Model file for the job. Use its own axes, mm. Face numbers are marked on the shaded views. A direction names the side the tool comes from. Give positions to 0.01 mm unless a question says otherwise; leave off trailing zeros. Write each loop counter-clockwise with the first axis right and the second up, starting at its lowest first coordinate (ties: lowest second). Pieces come first, ordered by that corner, then holes. Notation, with made-up numbers: (46, -25.5) - (53, -25.5) arc R18 ccw to (53, -7.5) - close; hole circle Ø10 at (31, 16.25). An arc over 180 degrees is marked (long way). One line per item, written item: value. Start each with the question number.
(1) Drop flat-ended pins along their axis: P1, Ø12, axis at y = 300, z = -22.5, coming from the -X side; P2, Ø4, axis at x = -13.5, z = -37, coming from the -Y side; P3, Ø3.5, axis at x = -26.99, z = -26.99, coming from the -Y side (1 decimal); P4, Ø12, axis at x = -19.5, z = -29.5, coming from the -Y side. Give the stop position or say it passes through.
(2) Cut at B-B, the plane y = 261. List the corners of the cut face in (x, z) (1 decimal).
(3) Cut at A-A, the plane y = 227. List the corners of the cut face in (x, z) (1 decimal).
(4) 3-axis set-ups, long thin cutter, end or side, ignore diameter. For the marked faces 1 and 2: which of +Z, -Z, +X, -X, +Y, -Y reach the whole face in a straight line?
(5) Cut at C-C, the plane x = -5. List the corners of the cut face in (y, z) (3 decimals), and give its area (3 significant figures).
(6) Probe L1, parallel to Y at x = -23.5, z = -38; L2, parallel to X at y = 248.5, z = -28.5; L3, parallel to Z at x = -28, y = 237. List the from-to ranges inside material, lowest first.
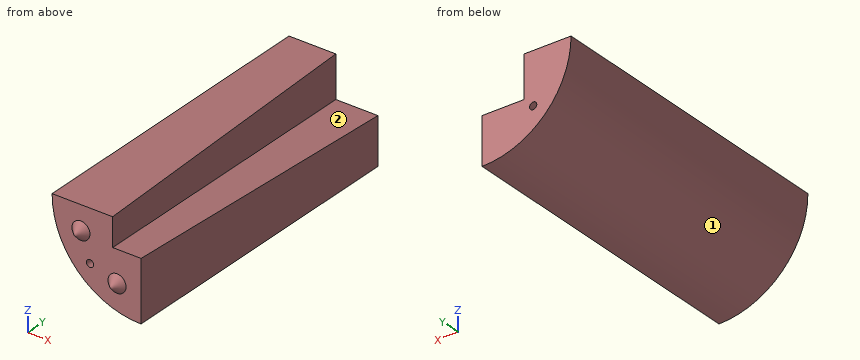
from build123d import *

# Parameters (mm, degrees)
SKETCH1_R           = 46.99
BOSS_EXTRUDE1_DEPTH = 330.2
SKETCH2_W           = 44.45
SKETCH2_H           = 44.45
CUT_EXTRUDE1_DEPTH  = 330.2
CUT_EXTRUDE1_DRAFT  = -2.5
CUT_EXTRUDE2_START  = -330.2
SKETCH3_R           = 1.905
CUT_EXTRUDE2_DEPTH  = 330.2
CUT_EXTRUDE3_DEPTH  = 165.1


with BuildPart() as part:
    # Sketch1 → Boss-Extrude1 (new body)
    with BuildSketch(Plane(origin=(0, 0, 0), x_dir=(1, 0, 0), z_dir=(0, 1, 0))):
        with Locations(Location((0, 0, 0), (0, 0, 270))):
            Circle(SKETCH1_R)
    extrude(amount=BOSS_EXTRUDE1_DEPTH)


with BuildPart() as cut_extrude1_tool:
    # Sketch2 → Cut-Extrude1 (with draft: the straight prism first)
    with BuildSketch(Plane(origin=(0, 330.2, 0), x_dir=(1, 0, 0), z_dir=(0, 1, 0))):
        Rectangle(SKETCH2_W, SKETCH2_H)
    extrude(amount=-CUT_EXTRUDE1_DEPTH)
    # Cut-Extrude1: the draft: its side faces are tilted about the plane it starts from
    cut_extrude1_sides = [cut_extrude1_tool.faces().sort_by_distance(p)[0] for p in [
        (-22.225, 165.1, 0),
        (0, 165.1, 22.225),
        (22.225, 165.1, 0),
        (0, 165.1, -22.225),
    ]]
    draft(cut_extrude1_sides, Plane(origin=(0, 330.2, 0), x_dir=(1, 0, 0), z_dir=(0, 1, 0)), CUT_EXTRUDE1_DRAFT)


with BuildPart() as part_1:
    add(part.part)

    # Cut-Extrude1: cut by cut_extrude1_tool
    add(cut_extrude1_tool.part, mode=Mode.SUBTRACT)

    # Sketch3 → Cut-Extrude2 (cut)
    with BuildSketch(Plane(origin=(0, 330.2, 0), x_dir=(1, 0, 0), z_dir=(0, 1, 0)).offset(CUT_EXTRUDE2_START)):
        with Locations(Location((-26.9875, 26.9875, 0), (0, 0, 270))):
            Circle(SKETCH3_R)
        with BuildLine():
            Line((0, 12.7), (0, 46.99))
            ThreePointArc((0, 46.99), (33.226947648, -33.226947648), (-46.99, 0))
            Line((-46.99, 0), (-12.7, 0))
            Line((-12.7, 0), (0, 0))
            Line((0, 0), (0, 12.7))
        make_face()
    extrude(amount=CUT_EXTRUDE2_DEPTH, mode=Mode.SUBTRACT)

    # Sketch5 → Cut-Extrude3 (cut)
    with BuildSketch(Plane.XZ):
        with BuildLine():
            Line((-46.99, 0), (0, 0))
            Line((0, 0), (0, -46.99))
            ThreePointArc((0, -46.99), (-33.226947648, -33.226947648), (-46.99, 0))
        make_face()
    extrude(amount=-CUT_EXTRUDE3_DEPTH, mode=Mode.SUBTRACT)

    # Boss-Extrude3 cone 1 section (through the dimple's axis) → Boss-Extrude3 (revolve)
    with BuildSketch(Plane(origin=(-31.75, 165.1, -12.7), x_dir=(0, 0, 1), z_dir=(1, 0, 0))):
        Polygon((0, 0), (4.7625, 0), (0, 4.7625), align=None)
    revolve(axis=Axis((-31.75, 165.1, -12.7), (0, -1, 0)))

    # Boss-Extrude3 cone 2 section (through the dimple's axis) → Boss-Extrude3 cone 2 (revolve)
    with BuildSketch(Plane(origin=(-12.7, 165.1, -31.75), x_dir=(0, 0, 1), z_dir=(1, 0, 0))):
        Polygon((0, 0), (4.7625, 0), (0, 4.7625), align=None)
    revolve(axis=Axis((-12.7, 165.1, -31.75), (0, -1, 0)))


solid = part_1.part
Answers follow:
1. P1: stops at x = -44
1. P2: stops at y = 163.65
1. P3: passes through
1. P4: stops at y = 161.5
2. outline: (-47, 0) arc R47 ccw to (0, -47) - (0, -19.2) - (-19.2, -19.2) - (-19.2, 0) - close; hole circle Ø3.8 at (-27, -27)
3. outline: (-47, 0) arc R47 ccw to (0, -47) - (0, -17.7) - (-17.7, -17.7) - (-17.7, 0) - close; hole circle Ø3.8 at (-27, -27)
4. face 1: -Z, -X, +Y, -Y
4. face 2: +Z, +X, +Y
5. outline: (165.1, -46.723) - (330.2, -46.723) - (330.2, -22.225) - (165.1, -15.017) - close
5. area: 4,640 mm²
6. L1: y = 165.1 to 330.2
6. L2: x = -37.36 to -28.15, -25.83 to 0
6. L3: z = -37.74 to -28.6, -25.37 to 0
